Design review of the part built by this model. Coordinates are the model's own, in mm. A direction names the side the tool comes from. Give positions to 0.01 mm unless a question says otherwise; leave off trailing zeros. Write each loop counter-clockwise with the first axis right and the second up, starting at its lowest first coordinate (ties: lowest second). Pieces come first, ordered by that corner, then holes. Notation, with made-up numbers: M 7.5,51.25 L 64.5,51.25 A22 ccw 64.5,78.25 Z; hole C 60,-8.75 d11. An arc over 180 degrees is marked long. Write each question's results on one line, items separated by ' | '. Start each with the question number.
Autodesk Inventor part; units mm, degrees
ref_plane "Work Plane1" through (0, 0, 0) normal (0, -1, 0) x (1, 0, 0)
ref_plane "YZ Plane" through (0, 0, 0) normal (1, 0, 0) x (0, 1, 0)
ref_plane "XZ Plane" through (0, 0, 0) normal (0, 1, 0) x (-1, 0, 0)
sketch "Sketch1" plane through (0, 0, 0) normal (1, 0, 0) x (0, 1, 0)
  circle A0 centre (0, 0) radius 6.2103
  circle A1 centre (0, 0) radius 3.2004
  dimension "d0" = 6.4008
  dimension "d1" = 12.4206
extrude "Body" add sketch "Sketch1" along normal blind 1.9558
sketch "Sketch2" plane through (0, 0, 0) normal (0, 0, 1) x (1, 0, 0)
  line L0 (0, -3.2004) -> (0, 3.2004)
  line L1 (1.9558, 6.2103) -> (1.9558, -6.2103)
  line L2 (-1.2, 0) -> (7.2, 0)
  line L3 (0, -0.3912) -> (1.9558, -0.3912)
  line L4 (0, 0.3912) -> (1.9558, 0.3912)
  dimension "d4" = 0.3912
  dimension "d5" = 0.3912
  dimension "d6" = 90
extrude "Cut" cut sketch "Sketch2" along normal up to next
ref_plane "Work Plane1" through (0, 0, 0) normal (0, -1, 0) x (1, 0, 0)
equation "\"d0\" = SD1"
equation "\"d1\" = SD2"
equation "\"d2\" = SD"
equation "\"d4\" = 0.2 * SD"
equation "\"d5\" = 0.2 * SD"
equation "\"d6\" = FAWI"
equation "\"d7\" = SD"
equation "\"SD1\" = 6.4008"
equation "\"SD2\" = 12.4206"
equation "\"SD\" = 1.9558"
equation "\"FAWI\" = 90deg"
equation "\"NND\" = 6.35"
properties part number "ASME B18.21.1 - 1/4" material "Steel, Mild"
Q1. We need section C-C on y = 0. Write out the cut boundary in (x, z).
Q2. The part is to be moulded in two halves that separate along Y. For faces 3 (the flat face through (1, 0.391, 5)), 4 (the flat face through (0, 3, -3)), say which applies: pulls with the +Y half, pulls with the -Y half, needs draft (parallel to the pull), parting line crosses it, or undercut.
Q3. For faces 1 (the flat face through (1, -0.391, 5)), 2 (the flat face through (1.956, 3, -3)), list the 3-axis set-ups (+Z, -Z, +X, -X, +Y, -Y) from which the entire face can be reached by the end or side of a thin tool; tool diameter is ignored.
Q4. For pin 1 Ø1 at (x, z) = (1, 5.5) entering from +Y, flat-tipped, find the tip position at first contact; note if it passes through.
Q5. We need section B-B on x = 0.5. Write out the cut boundary in (y, z), and give its area (3 significant figures).
Q6. We need section A-A on z = -1.5. Write out the cut boundary in (x, y), and give its area (3 significant figures).
Q7. We need section D-D on z = 2. Write out the cut boundary in (x, y).
Q8. Wall thickness on line 1 along Y through (x, z) = (0.8, 0); line 2 along Y through (x, z) = (1.7, 2); line 3 along Z through (x, y) = (1.1, 0): over which ranges is each line inside the solid? List them lowest first. Write a range as from..to.
Answer sheet:
1) outline: M 0,-6.21 L 1.96,-6.21 L 1.96,-3.2 L 0,-3.2 Z
2) face 3: undercut | face 4: needs draft
3) face 1: +Z, +X, -X | face 2: +Z, -Z, +X, +Y, -Y
4) pin 1: y = 3.68
5) outline: M -0.39,3.18 L -0.39,6.2 A6.21 ccw long 0.39,6.2 L 0.39,3.18 A3.2 cw long Z | area: 86.6 mm^2
6) outline: M 0,-6.03 L 1.96,-6.03 L 1.96,-2.83 L 0,-2.83 Z; M 0,2.83 L 1.96,2.83 L 1.96,6.03 L 0,6.03 Z | area: 12.5 mm^2
7) outline: M 0,-5.88 L 1.96,-5.88 L 1.96,-2.5 L 0,-2.5 Z; M 0,2.5 L 1.96,2.5 L 1.96,5.88 L 0,5.88 Z
8) line 1: -6.21..-3.2, 3.2..6.21 | line 2: -5.88..-2.5, 2.5..5.88 | line 3: -6.21..-3.2
